```python
from build123d import *


# Not quite as in the source:
# - a feature names something its author has since deleted; it is built from what else it names


with BuildPart() as f1:
    # F0 (on Front) → F1 (revolve)
    with BuildSketch(Plane.XZ):
        with BuildLine():
            Line((0, 480), (0, 0))
            Line((0, 0), (0, -480))
            Line((0, -480), (17, -480))
            Line((17, -480), (25.7319285466, -102.9642244203))
            ThreePointArc((25.7319285466, -102.9642244203), (25.9329798908, -91.3883962972), (26, -79.8110163396))
            Line((26, -79.8110163396), (26, 0))
            Line((26, 0), (26, 79.8110163396))
            ThreePointArc((26, 79.8110163396), (25.9329798908, 91.3883962972), (25.7319285466, 102.9642244203))
            Line((25.7319285466, 102.9642244203), (17, 480))
            Line((17, 480), (0, 480))
        make_face()
    revolve(axis=Axis((0, 0, 240), (0, 0, 1)))


solid = f1.part
```
The listing builds one solid part. Answer for the finished solid, in the listing's coordinates (mm). A direction names the side the tool comes from. Coordinates: 2 decimals unless noted, no trailing zeros. Write each loop counter-clockwise with the first axis right and the second up, starting at its lowest first coordinate (ties: lowest second). Pieces come first, ordered by that corner, then holes. Notation, with made-up numbers: (-38.75, 68.25) - (-13.75, 68.25) arc R34 cw to (-13.75, 104.25) - close; hole circle Ø3 at (52, 6). An arc over 180 degrees is marked (long way). Return JSON: item names as keys, results as strings. Group by question number.
1. Straight lines are drawn through the part: L1, parallel to X at y = -17.5, z = -88; L2, parallel to Y at x = 4, z = -116.5; L3, parallel to X at y = -11, z = -426. For each, find the intervals that lie inside material, in ascending order.
2. A cutting plane is placed at B-B, the plane z = -210.5. Determine the outline of the cut face in (x, y), plus the area to 3 significant figures.
3. A cutting plane is placed at A-A, the plane z = -325. Determine the outline of the cut face in (x, y), plus the area to 3 significant figures.
4. Which of the six approach directions +Z, -Z, +X, -X, +Y, -Y give full straight-line access (tool end or side, diameter ignored) to faces 1 (the conical face through (-4.618, -20.798, 294.121)), 2 (the cylindrical face through (24.8, 7.81, 1.12)), 3 (the conical face through (-17, -13.04, -288.84))?
5. Given pin 1 (3 mm diameter, centred on x = 0.5, z = -228, fed in from -Y); pin 2 (8 mm diameter, centred on y = 18, z = 252, fed in from -X); pin 3 (5 mm diameter, centred on x = -17.5, z = -125.5, fed in from +Y), each flat-ended and moving along its own axis, determine where each tip first touches the part or whether it passes through.
Ans:
{
 "1": {"L1": "-19.18 to 19.18", "L2": "-25.1 to 25.1", "L3": "-14.56 to 14.56"},
 "2": {"outline": "circle Ø46.48 at (0, 0)", "area": "1,700 mm²"},
 "3": {"outline": "circle Ø41.18 at (0, 0)", "area": "1,330 mm²"},
 "4": {"face 1": "+Z", "face 2": "+Z, -Z", "face 3": "-Z"},
 "5": {"pin 1": "y = -22.87", "pin 2": "x = -17.33", "pin 3": "y = 20.26"}
}
